```python
from build123d import *

# Parameters (mm, degrees)
SKETCH1_W           = 114.3
SKETCH1_H           = 19.05
BOSS_EXTRUDE1_DEPTH = 3.175
FILLET1_R           = 19.05


with BuildPart() as part:
    # Sketch1 → Boss-Extrude1 (new body)
    with BuildSketch(Plane(origin=(0, 0, 0), x_dir=(0, 0, -1), z_dir=(1, 0, 0))):
        Rectangle(SKETCH1_W, SKETCH1_H)
    extrude(amount=BOSS_EXTRUDE1_DEPTH)

    # Fillet1
    fillet1_edges = [part.edges().sort_by_distance(p)[0] for p in [
        (1.5875, 9.525, -57.15),
        (1.5875, 9.525, 57.15),
    ]]
    fillet(fillet1_edges, radius=FILLET1_R - 0.0001)  # a hair under: the kernel refuses the full size


solid = part.part
```
Input: part model. Units: mm. Frame: model coordinates. Round coordinates to 2 decimals unless told otherwise and drop trailing zeros. Loops run counter-clockwise (first coordinate to the right, second up) from the corner with the lowest first, then second, coordinate; pieces in that order, holes last. Notation, with made-up numbers: (-12.5, -32.5) -> (34.5, -32.5) arc R7 cw to (34.5, -26.5) -> close; hole circle Ø10 at (61, 46). An arc over 180 degrees is marked (long way). Use one line per item in the form item = value. Start each with the question number.
Item 1: Section query C-C on z = 43.5. Return the cut outline in (x, y) (3 decimals).
Item 2: Material intervals for L1, parallel to Z at x = 0.75, y = -2.25; L2, parallel to Y at x = 1.55, z = 38.5 (3 decimals); L3, parallel to Z at x = 1.8, y = -4.75, sorted ascending. Write a range as from..to.
Item 3: Section query B-B on y = -2. Return the cut outline in (x, z) (3 decimals).
Ans:
q1.outline = (0, -9.525) -> (3.175, -9.525) -> (3.175, 8.744) -> (0, 8.744) -> close
q2.L1 = -55.71..55.71
q2.L2 = -9.525..9.521
q2.L3 = -56.54..56.54
q3.outline = (0, -55.601) -> (3.175, -55.601) -> (3.175, 55.601) -> (0, 55.601) -> close
